Part print with two shaded views. Sizes in mm from the minimum x, y, z corner. Round coordinates to 2 decimals unless told otherwise and drop trailing zeros. Write each loop counter-clockwise with the first axis right and the second up, starting at its lowest first coordinate (ties: lowest second). Pieces come first, ordered by that corner, then holes. Notation, with made-up numbers: (42, -29.75) - (100, -29.75) arc R34 ccw to (100, 0.25) - close; hole circle Ø6 at (-1, 54). An arc over 180 degrees is marked (long way). Answer as a JSON object with one key per item and string values. Group by question number.
Item 1: Slice it at B-B, the plane z = 5.5. Give the number of separate pieces and of enclosed holes in the cut face, then the cut area to 3 significant figures.
Item 2: Slice it at A-A, the plane x = 50. List the corners of the cut face in (y, z).
Item 3: Probe line 1 (Y direction, x = 199, z = 4.25); line 2 (Y direction, x = 200, z = 5); line 3 (Y direction, x = 350, z = 5.75). List the from-to ranges inside material, lowest first. Write a range as from..to.
Item 4: Slice it at D-D, the plane x = 200. List the corners of the cut face in (y, z), then the cut area to 3 significant figures.
Item 5: Flat gauge pins, fed straight in: pin 1 (4 mm diameter, centred on x = 218.5, y = 99.5, fed in from -Z); pin 2 (3.5 mm diameter, centred on y = 279.5, z = 5, fed in from -X). Where does each tip first touch, or does it go through?
Item 6: Slice it at C-C, the plane y = 50. List the corners of the cut face in (x, z), then the cut area to 3 significant figures.
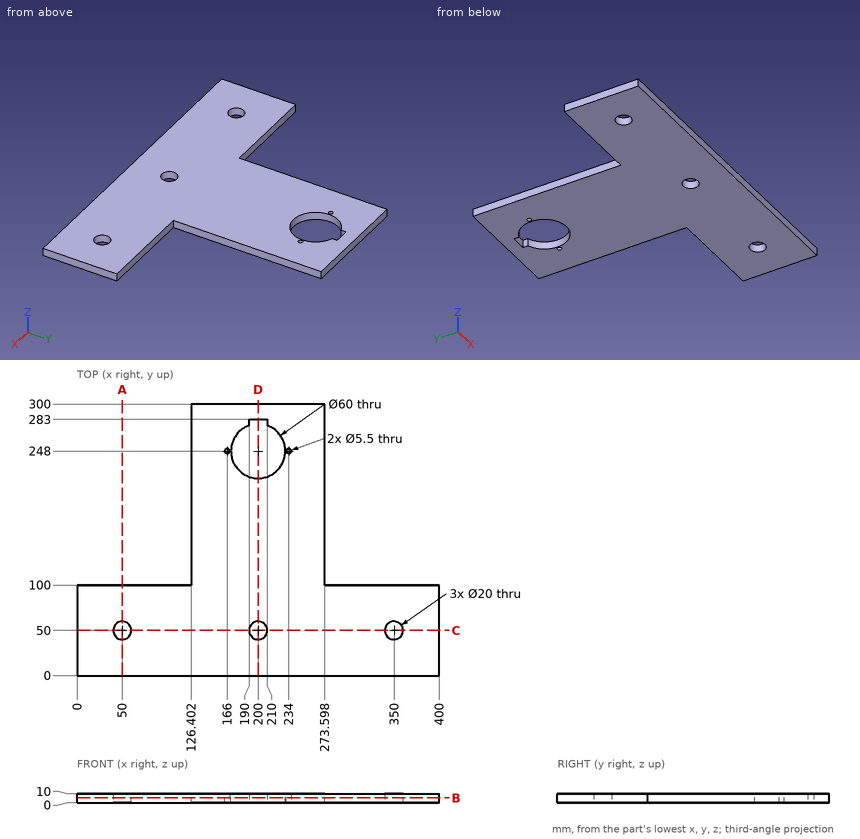
Geometry says:
{
 "1": {"separate pieces": "1", "enclosed holes": "6", "area": "65,500 mm^2"},
 "2": {"outline": "(0, 0) - (40, 0) - (40, 10) - (0, 10) - close; (60, 0) - (100, 0) - (100, 10) - (60, 10) - close"},
 "3": {"line 1": "y = 0..40.05, 59.95..218.02, 283..300", "line 2": "y = 0..40, 60..218, 283..300", "line 3": "y = 0..40, 60..100"},
 "4": {"outline": "(0, 0) - (40, 0) - (40, 10) - (0, 10) - close; (60, 0) - (218, 0) - (218, 10) - (60, 10) - close; (283, 0) - (300, 0) - (300, 10) - (283, 10) - close", "area": "2,150 mm^2"},
 "5": {"pin 1": "stops at z = 0", "pin 2": "stops at x = 126.4"},
 "6": {"outline": "(0, 0) - (40, 0) - (40, 10) - (0, 10) - close; (60, 0) - (190, 0) - (190, 10) - (60, 10) - close; (210, 0) - (340, 0) - (340, 10) - (210, 10) - close; (360, 0) - (400, 0) - (400, 10) - (360, 10) - close", "area": "3,400 mm^2"}
}
